```python
from build123d import *

# Parameters (mm, degrees)
SKETCH1_W             = 5.95
SKETCH1_H             = 5.95
BOSS_EXTRUDE1_DEPTH   = 0.1
BOSS_EXTRUDE2_START   = 0.1
SKETCH2_W             = 6
SKETCH2_H             = 6
BOSS_EXTRUDE2_DEPTH   = 2.9
FILLET1_R             = 0.1
BOSS_EXTRUDE3_START   = -0.1
SKETCH3_R             = 1.65
SKETCH3_R_2           = 0.55
BOSS_EXTRUDE3_DEPTH   = 0.2
BOSS_EXTRUDE4_START   = -0.1
SKETCH4_R             = 1.65
BOSS_EXTRUDE4_DEPTH   = 1
BODY_MOVE_COPY1_ANGLE = 179.5


with BuildPart() as part:
    # Sketch1 → Boss-Extrude1 (new body, symmetric)
    with BuildSketch(Plane.XY):
        with Locations((-2.975, -2.975)):
            Rectangle(SKETCH1_W, SKETCH1_H)
    extrude(amount=BOSS_EXTRUDE1_DEPTH, both=True)

    # Sketch2 → Boss-Extrude2 (add)
    with BuildSketch(Plane.XY.offset(BOSS_EXTRUDE2_START)):
        with Locations((-2.975, -2.975)):
            Rectangle(SKETCH2_W, SKETCH2_H)
    extrude(amount=BOSS_EXTRUDE2_DEPTH)

    # Fillet1
    fillet1_edges = [part.edges().sort_by_distance(p)[0] for p in [
        (0, -5.95, 0),
        (-5.95, -5.95, 0),
        (-5.95, 0, 0),
        (0, 0, 0),
    ]]
    fillet(fillet1_edges, radius=FILLET1_R)

    # Sketch3 → Boss-Extrude3 (add)
    with BuildSketch(Plane.XY.offset(BOSS_EXTRUDE3_START)):
        with Locations((-2.975, -2.975)):
            Circle(SKETCH3_R)
        with Locations((-5.075, -0.875)):
            Circle(SKETCH3_R_2)
        with Locations((-5.075, -5.075)):
            Circle(SKETCH3_R_2)
        with Locations((-0.875, -5.075)):
            Circle(SKETCH3_R_2)
        with Locations((-0.875, -0.875)):
            Circle(SKETCH3_R_2)
    extrude(amount=-BOSS_EXTRUDE3_DEPTH)

    # Sketch4 → Boss-Extrude4 (add)
    with BuildSketch(Plane.XY.offset(BOSS_EXTRUDE4_START)):
        with Locations((-2.975, -2.975)):
            Circle(SKETCH4_R)
    extrude(amount=-BOSS_EXTRUDE4_DEPTH)


with BuildPart() as part_1:
    # Body-Move/Copy1: moved
    add(part.part.rotate(Axis((-2.975, 0, 0.95), (0, -1, 0)), BODY_MOVE_COPY1_ANGLE))


solid = part_1.part
```
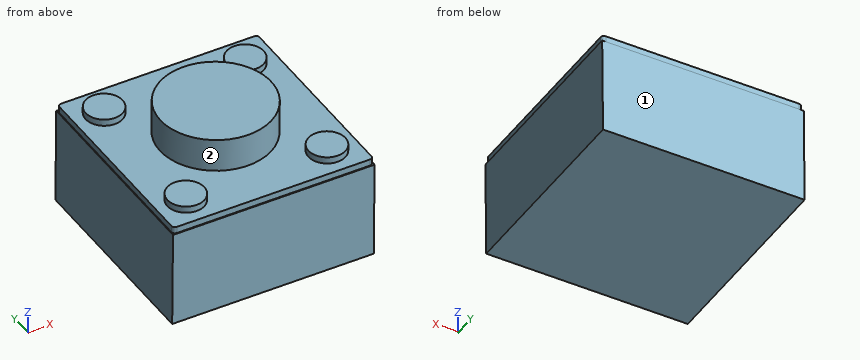
The model under review builds one solid part; all positions refer to its coordinate system, in mm. Face numbers are marked on the shaded views. A direction names the side the tool comes from. Round coordinates to 2 decimals unless told otherwise and drop trailing zeros. Use CSV: the item, a comma, the result in double quotes. Start each with the question number.
(1) Clearance check with flat-ended pins moving along their axes: P1, Ø1, axis at y = -4.5, z = -0.5, coming from the +X side; P2, Ø2, axis at x = -4, y = -2.5, coming from the +Z side. State where each tip first meets the part, or that it passes through.
(2) Tool access review of the marked faces 1 and 2: name each direction out of +Z, -Z, +X, -X, +Y, -Y from which nothing blocks a thin tool from reaching the whole face with its end or side.
(3) For line 1 along X through (y, z) = (-0.5, 1.9); line 2 along X through (y, z) = (-2.7, 1.2); line 3 along Z through (x, y) = (-2, -1.6), list the stretches that pass through material, from the lowest coordinate up.
Findings:
1,P1,"x = 0.02"
1,P2,"z = 3.01"
2,face 1,"+Z, -Z, +X, -X, +Y"
2,face 2,"none"
3,line 1,"-5.94 to 0.01"
3,line 2,"-5.97 to 0.03"
3,line 3,"-1.11 to 1.99"
